Geometry: see drawing. Coordinates: mm, zero at the bounding-box minimum. A direction names the side the tool comes from. Give positions to 0.01 mm unless a question says otherwise; leave off trailing zeros. Write each loop counter-clockwise with the first axis right and the second up, starting at its lowest first coordinate (ties: lowest second). Pieces come first, ordered by that corner, then holes. Notation, with made-up numbers: (63.25, -37.5) -> (90.25, -37.5) arc R26 cw to (90.25, 1.5) -> close; hole circle Ø1 at (-22, 81). An arc over 180 degrees is marked (long way). Answer as a JSON object with one key per item and string values. Group by question number.
Item 1: Section query A-A on z = 4.5. Return the cut outline in (x, y).
Item 2: Access query for the marked faces 1, 2, 3, 4 and 5. Directions: +Z, -Z, +X, -X, +Y, -Y. A direction counts if a zero-diameter tool reaches every point of the face in a straight line with its end or side. Return the directions, or none.
Item 3: Ray query, probe 1 along X at (y, z) = (1.5, 0.5); probe 2 along Y at (x, z) = (41, 2.5). Return the intervals inside material, ascending. Write a range as from..to.
Item 4: First-contact query: pin 1 Ø1.5 at (x, z) = (13, 5.5) entering from -Y; pin 2 Ø3 at (x, y) = (42, 3) entering from +Z; pin 3 Ø3 at (x, y) = (5, 4) entering from -Z. Flat tips, straight axial feed; report the tip coordinate or a pass-through.
Item 5: Section query C-C on x = 10.5. Return the cut outline in (y, z).
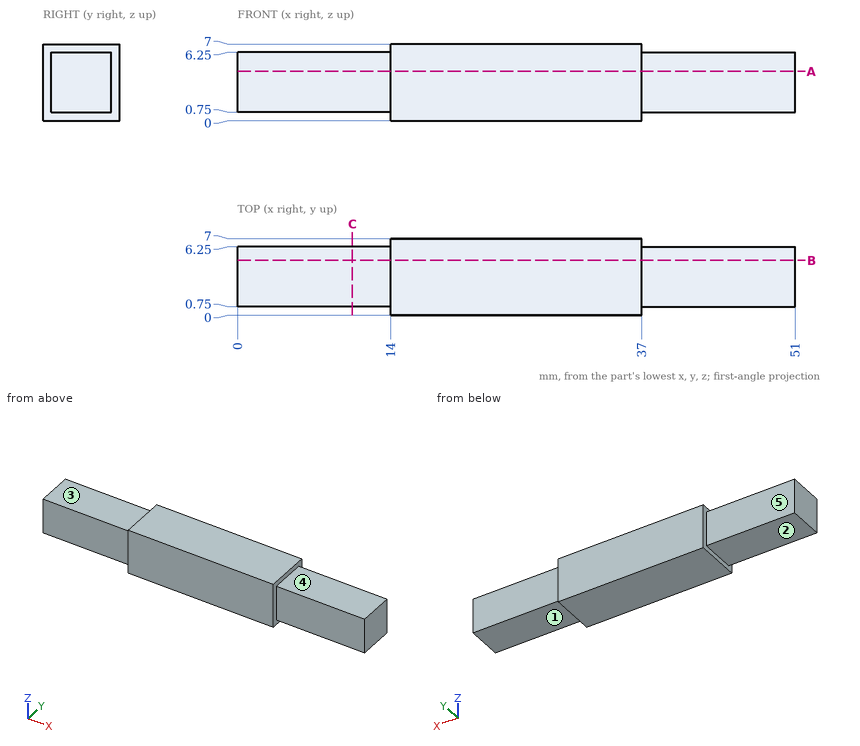
Worked answers:
{
 "1": {"outline": "(0, 0.75) -> (14, 0.75) -> (14, 0) -> (37, 0) -> (37, 0.75) -> (51, 0.75) -> (51, 6.25) -> (37, 6.25) -> (37, 7) -> (14, 7) -> (14, 6.25) -> (0, 6.25) -> close"},
 "2": {"face 1": "-Z, +X, +Y, -Y", "face 2": "-Z, -X, +Y, -Y", "face 3": "+Z, -X, +Y, -Y", "face 4": "+Z, +X, +Y, -Y", "face 5": "+Z, -Z, -X, +Y"},
 "3": {"probe 1": "14..37", "probe 2": "0.75..6.25"},
 "4": {"pin 1": "y = 0.75", "pin 2": "z = 6.25", "pin 3": "z = 0.75"},
 "5": {"outline": "(0.75, 0.75) -> (6.25, 0.75) -> (6.25, 6.25) -> (0.75, 6.25) -> close"}
}
